Here's how the part is built. I have some questions about the finished solid (model axes, mm). Face numbers are marked on the shaded views. A direction names the side the tool comes from. Coordinates: 2 decimals unless noted, no trailing zeros. Write each loop counter-clockwise with the first axis right and the second up, starting at its lowest first coordinate (ties: lowest second). Pieces come first, ordered by that corner, then holes.
Item 1: If we section it at C-C (y = -7): Please give me the cut outline in (x, z).
Item 2: If I drill on line 1 (Y direction, x = 58, z = -4.25); line 2 (X direction, y = 0.75, z = -2.75); line 3 (Z direction, x = 84.5, y = -1), over which ranges is the centre line in solid material (lowest first)?
Item 3: For the marked faces 1 and 2, which set-ups out of +Z, -Z, +X, -X, +Y, -Y let a thin tool reach every point of the face, with its end or its side?
Item 4: I'm going to push flat-ended pins straight in: pin 1 Ø1.5 at (y, z) = (-3.5, -1.5) entering from -X; pin 2 Ø2 at (y, z) = (-6, 1) entering from +X; pin 3 Ø6 at (x, z) = (-14.57, -1.71) entering from -Y. Where does each tip first touch, or does it pass through?
Item 5: If we section it at B-B (x = 26): Please give me the cut outline in (y, z).
Item 6: If we section it at A-A (y = 2.5): Please give me the cut outline in (x, z), then the cut area to 3 significant figures.
from build123d import *

# Parameters (mm, degrees)
SKETCH1_R           = 2.5
BOSS_EXTRUDE1_DEPTH = 5
SKETCH2_R           = 2.5
BOSS_EXTRUDE2_DEPTH = 15


with BuildPart() as part:
    # Sketch1 → Boss-Extrude1 (new body)
    with BuildSketch(Plane(origin=(0, 0, 0), x_dir=(1, 0, 0), z_dir=(0, 1, 0))):
        with BuildLine():
            Line((-14.504443595, 6.706697569), (85.495556405, 5.363127511))
            ThreePointArc((85.495556405, 5.363127511), (90.42793273, 0.296406305), (85.361211524, -4.635970021))
            Line((85.361211524, -4.635970021), (-14.638788476, -3.292399963))
            ThreePointArc((-14.638788476, -3.292399963), (-19.571164802, 1.774321243), (-14.504443595, 6.706697569))
        make_face()
        with Locations(Location((-14.571616036, 1.707148803, 0), (0, 0, 270))):
            Circle(SKETCH1_R, mode=Mode.SUBTRACT)
    extrude(amount=BOSS_EXTRUDE1_DEPTH)

    # Sketch2 → Boss-Extrude2 (add)
    with BuildSketch(Plane(origin=(0, 5, 0), x_dir=(1, 0, 0), z_dir=(0, 1, 0))):
        with Locations(Location((85.428383964, 0.363578745, 0), (0, 0, 270))):
            Circle(SKETCH2_R)
    extrude(amount=-BOSS_EXTRUDE2_DEPTH)


solid = part.part
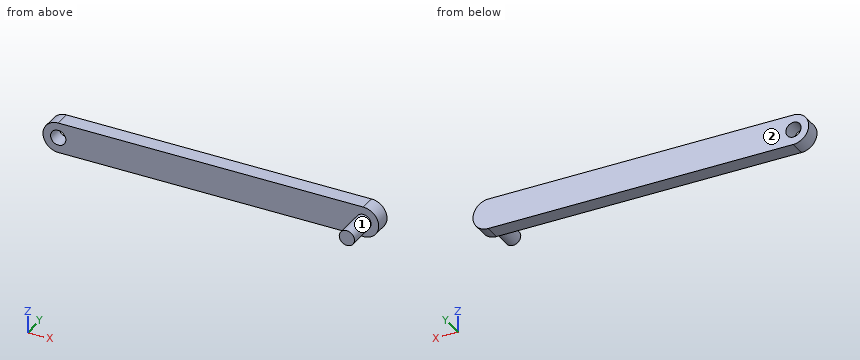
Answer list:
1. outline: circle Ø5 at (85.43, -0.36)
2. line 1: y = 0 to 5
2. line 2: x = -19.46 to -16.84, -12.3 to 89.82
2. line 3: z = -2.68 to 1.96
3. face 1: -Y
3. face 2: +Z, -Z, +X, -X, +Y
4. pin 1: stops at x = 82.96
4. pin 2: stops at x = 87.9
4. pin 3: stops at y = 0
5. outline: (0, -6.16) - (5, -6.16) - (5, 3.84) - (0, 3.84) - close
6. outline: (-14.64, 3.29) arc R5 ccw to (-14.5, -6.71) - (85.5, -5.36) arc R5 ccw to (85.36, 4.64) - close; hole circle Ø5 at (-14.57, -1.71)
6. area: 1,060 mm2
